```python
from build123d import *

# Parameters (mm, degrees)
CYLINDER458_R     = 1.6
CYLINDER458_DEPTH = 15
CYLINDER459_R     = 1.6
CYLINDER459_DEPTH = 15
BOX311_W          = 34
BOX311_H          = 12
BOX311_DEPTH      = 20
FILLET111_R       = 3
BOX310_W          = 34
BOX310_H          = 12
BOX310_DEPTH      = 24


with BuildPart() as cylinder458:
    # Cylinder458 → Cylinder458 (new body)
    with BuildSketch(Plane(origin=(588, 6, 10), x_dir=(1, 0, 0), z_dir=(0, -1, 0))):
        Circle(CYLINDER458_R)
    extrude(amount=CYLINDER458_DEPTH)


with BuildPart() as fusion415:
    # Cylinder459 → Cylinder459 (new body)
    with BuildSketch(Plane(origin=(570, 6, 10), x_dir=(1, 0, 0), z_dir=(0, -1, 0))):
        Circle(CYLINDER459_R)
    extrude(amount=CYLINDER459_DEPTH)

    # Fusion415: union Cylinder458
    add(cylinder458.part)


with BuildPart() as fusion415_1:
    # Fusion415 placement: moved
    add(fusion415.part.moved(Location((0, -4, 0))))


with BuildPart() as fillet111:
    # Box311 → Box311 (new body)
    with BuildSketch(Plane(origin=(565, -9, 0), x_dir=(1, 0, 0), z_dir=(0, 0, 1))):
        with Locations((17, 6)):
            Rectangle(BOX311_W, BOX311_H)
    extrude(amount=BOX311_DEPTH)

    # Fillet111
    fillet111_edges = [fillet111.edges().sort_by_distance(p)[0] for p in [
        (582, -9, 0),
        (582, -9, 20),
    ]]
    fillet(fillet111_edges, radius=FILLET111_R)


with BuildPart() as rear_cross_member_wide_holes:
    # Box310 → Box310 (new body)
    with BuildSketch(Plane(origin=(565, -11, -2), x_dir=(1, 0, 0), z_dir=(0, 0, 1))):
        with Locations((17, 6)):
            Rectangle(BOX310_W, BOX310_H)
    extrude(amount=BOX310_DEPTH)

    # Cut308: cut Fillet111
    add(fillet111.part, mode=Mode.SUBTRACT)

    # Cut309: cut Fusion415
    add(fusion415_1.part, mode=Mode.SUBTRACT)


solid = rear_cross_member_wide_holes.part
```
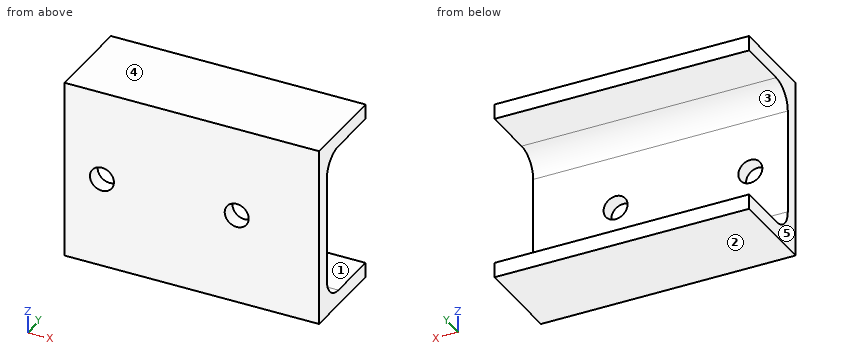
Here's how the part is built. I have some questions about the finished solid (model axes, mm). Face numbers are marked on the shaded views. A direction names the side the tool comes from. Give positions to 0.01 mm unless a question says otherwise; leave off trailing zeros. Loops run counter-clockwise (first coordinate to the right, second up) from the corner with the lowest first, then second, coordinate; pieces in that order, holes last. Notation, with made-up numbers: (14, 26) -> (42, 26) arc R24 ccw to (42, 41) -> close; hole circle Ø1 at (51, -3.75). An arc over 180 degrees is marked (long way). Use one line per item in the form item = value. Start each with the question number.
1) Imagine slicing it at C-C (z = 10). Please give me the cut outline in (x, y), then the cut area to 3 significant figures.
2) Thinking about a two-plate mould opening in Z: for the marked faces 3, 4 and 5, which applies, +Z half, -Z half, draft (parallel to the pull), parting line (faces both ways), or undercut?
3) Imagine slicing it at D-D (x = 585). Please give me the cut outline in (y, z).
4) Imagine slicing it at A-A (y = -5). Please give me the cut outline in (x, z), then the cut area to 3 significant figures.
5) Imagine slicing it at B-B (x = 570). Please give me the cut outline in (y, z), then the cut area to 3 significant figures.
6) Which directions (+Z, -Z, +X, -X, +Y, -Y) give clear straight access to the entire face, cutting with the end or side of a thin tool? Please do the marked faces 1 and 2.
7) Please list where these lines run through material, in increasing order: line 1 along X through (y, z) = (-10.3, 10); line 2 along Z through (x, y) = (582, -5); line 3 along Z through (x, y) = (588, -10.25).
8) For P1, Ø10, axis at x = 594.5, z = 8.5, coming from the +Y side; P2, Ø2.5, axis at x = 570, z = 10, coming from the -Y side, each with a flat end and sliding along its axis, tell me the tip position at first contact or that it passes through.
Check values:
q1.outline = (565, -11) -> (568.4, -11) -> (568.4, -9) -> (565, -9) -> close; (571.6, -11) -> (586.4, -11) -> (586.4, -9) -> (571.6, -9) -> close; (589.6, -11) -> (599, -11) -> (599, -9) -> (589.6, -9) -> close
q1.area = 55.2 mm^2
q2.face_3 = undercut
q2.face_4 = +Z half
q2.face_5 = draft
q3.outline = (-11, -2) -> (1, -2) -> (1, 0) -> (-6, 0) arc R3 cw to (-9, 3) -> (-9, 17) arc R3 cw to (-6, 20) -> (1, 20) -> (1, 22) -> (-11, 22) -> close
q4.outline = (565, -2) -> (599, -2) -> (599, 0) -> (565, 0) -> close; (565, 20) -> (599, 20) -> (599, 22) -> (565, 22) -> close
q4.area = 136 mm^2
q5.outline = (-11, -2) -> (1, -2) -> (1, 0) -> (-6, 0) arc R3 cw to (-9, 3) -> (-9, 8.4) -> (-11, 8.4) -> close; (-11, 11.6) -> (-9, 11.6) -> (-9, 17) arc R3 cw to (-6, 20) -> (1, 20) -> (1, 22) -> (-11, 22) -> close
q5.area = 85.5 mm^2
q6.face_1 = +X, -X, +Y
q6.face_2 = -Z, +X, -X, +Y, -Y
q7.line_1 = 565 to 568.4, 571.6 to 586.4, 589.6 to 599
q7.line_2 = -2 to 0, 20 to 22
q7.line_3 = -2 to 8.4, 11.6 to 22
q8.P1 = -9
q8.P2 = through
